Autodesk Inventor part; units mm, degrees
ref_plane "YZ Plane" through (0, 0, 0) normal (1, 0, 0) x (0, 1, 0)
ref_plane "XZ Plane" through (0, 0, 0) normal (0, 1, 0) x (-1, 0, 0)
ref_plane "XY Plane" through (0, 0, 0) normal (0, 0, 1) x (1, 0, 0)
sketch "Sketch1" plane through (0, 0, 0) normal (0, 0, 1) x (1, 0, 0)
  line L0 (0, 0) -> (0, 15.875)
  line L1 (0, 15.875) -> (0.7937, 15.875)
  line L2 (0.7937, 15.875) -> (0.7938, 0.7937)
  line L3 (0.7938, 0.7937) -> (15.875, 0.7937)
  line L4 (15.875, 0.7937) -> (15.875, 0)
  line L5 (15.875, 0) -> (0, 0)
  dimension "d0" = 15.875
  dimension "d1" = 0.7937
extrude "Extrusion1" add sketch "Sketch1" along normal blind 82.55
sketch "Sketch2" plane through (0.7938, 0.7937, 0) normal (0, 1, 0) x (1, 0, 0)
  line L0 (0, 0) -> (15.0812, 0)
  line L1 (15.0812, -82.55) -> (0, -82.55)
  line L2 (7.5406, 0) -> (7.5406, -82.55) construction
  circle A0 centre (7.5406, -9.525) radius 1.5875
  circle A1 centre (7.5406, -73.025) radius 1.5875
  point P0 (-0.7938, 0)
  dimension "d4" = 9.525
  dimension "d5" = 3.175
  dimension "d6" = 82.55
  dimension "d9" = 63.5
sketch "Sketch3" plane through (0.7938, 0.7937, 0) normal (1, 0, 0) x (0, 0, -1)
  line L0 (0, 15.0812) -> (0, 0)
  line L1 (-82.55, 0) -> (-82.55, 15.0812)
  line L2 (-82.55, 7.5406) -> (0, 7.5406) construction
  circle A0 centre (-9.525, 7.5406) radius 1.5875
  circle A1 centre (-73.025, 7.5406) radius 1.5875
  point P0 (0, -0.7937)
  dimension "d14" = 3.175
  dimension "d15" = 9.525
  dimension "d16" = 82.55
  dimension "d19" = 63.5
extrude "Extrusion2" cut sketch "Sketch2" against normal through all
extrude "Extrusion3" cut sketch "Sketch3" against normal through all
properties part number "Hopper Bracing Back Left P12" material "Aluminum 6061"
Design review of the part built by this model. Coordinates are the model's own, in mm. Coordinates: 2 decimals unless noted, no trailing zeros. Loops run counter-clockwise (first coordinate to the right, second up) from the corner with the lowest first, then second, coordinate; pieces in that order, holes last. Notation, with made-up numbers: (-25, 36) - (21, 36) arc R14 ccw to (21, 43) - close; hole circle Ø10 at (54, 53.5). An arc over 180 degrees is marked (long way). Use CSV: the item, a comma, the result in double quotes. Start each with the question number.
1. To check wall thickness, follow probe 1 along Y at (x, z) = (8.75, 22). State the ranges of the line that lie inside material, in increasing order.
2. Mouldability with a two-part tool opening along X and no side actions: class faces 1 (the cylindrical face through (6.75, 0.4, 9.46)), 2 (the flat face through (8, 0.794, 41)), 3 (the flat face through (0, 8, 41)) as released by +X, released by -X, zero draft, split by the parting line, or undercut.
3. Add section B-B on x = 5. Give the boundary of the cut face in (y, z).
4. Clearance check with flat-ended pins moving along their axes: pin 1 (2 mm diameter, centred on y = 7, z = 21, fed in from -X); pin 2 (3 mm diameter, centred on x = 8.33, z = 73.03, fed in from +Y); pin 3 (2 mm diameter, centred on x = 12.5, z = 32.5, fed in from +Y); pin 4 (6 mm diameter, centred on y = 9, z = 28.5, fed in from +X). State where each tip first meets the part, or that it passes through.
5. Add section A-A on z = 47. Give the boundary of the cut face in (x, y) (3 decimals), plus the area to 3 significant figures.
Resolved:
1,probe 1,"0 to 0.79"
2,face 1,"undercut"
2,face 2,"zero draft"
2,face 3,"released by -X"
3,outline,"(0, 0) - (0.79, 0) - (0.79, 82.55) - (0, 82.55) - close"
4,pin 1,"x = 0"
4,pin 2,"through"
4,pin 3,"y = 0.79"
4,pin 4,"x = 0.79"
5,outline,"(0, 0) - (15.875, 0) - (15.875, 0.794) - (0.794, 0.794) - (0.794, 15.875) - (0, 15.875) - close"
5,area,"24.6 mm2"
